Verification items for the finished model (mm, model axes). A direction names the side the tool comes from. Coordinates: 2 decimals unless noted, no trailing zeros. Loops run counter-clockwise (first coordinate to the right, second up) from the corner with the lowest first, then second, coordinate; pieces in that order, holes last. Notation, with made-up numbers: (-17.5, 19) - (-3.5, 19) arc R15 ccw to (-3.5, 23) - close; hole circle Ø6 at (20.25, 46.5). An arc over 180 degrees is marked (long way). One line per item, written item: value. Start each with the question number.
(1) Section check D-D (z = 0.5). Record the boundary of the cut face in (x, y).
(2) Gauge pin test, flat ends, axial feed: P1, Ø2.5, axis at x = 0, z = -12.75, coming from the +Y side; P2, Ø0.9, axis at x = 0, z = 12.75, coming from the +Y side; P3, Ø1.1, axis at x = -6.5, y = -0.5, coming from the +Z side; P4, Ø1.2, axis at y = -1, z = 9, coming from the -X side. Record the tip position at first contact, or that the pin passes through.
(3) Section check C-C (y = -0.9). Count the separate pieces of the cut face and the enclosed holes in it, plus the area to 3 significant figures.
(4) Section check B-B (x = 7.5). Record the boundary of the cut face in (y, z), plus the area to 3 significant figures.
(5) Set-up check for faces 5 (the face through (-4, 0, -9)), 6 (the face through (0, 0, -7.5)), 7 (the face through (5, -0.5, 0)): record each of +Z, -Z, +X, -X, +Y, -Y from which the full face is reachable in a straight line by a thin tool's end or side.
(6) Draft check along Z on faces 1 (the face through (0, 0, -11.5)), 2 (the face through (5, 0, -5)), 3 (the face through (9.859, -0.028, 2.797)), 4 (the face through (4, 0, -10)). Enter one of: +Z half, -Z half, draft (parallel to the pull), parting line (faces both ways), or undercut.
(7) Section check A-A (z = -10.75). Record the boundary of the cut face in (x, y), plus the area to 3 significant figures.
(8) Thickness scan on probe 1 along X at (y, z) = (-1, 0); probe 2 along X at (y, z) = (0.4, 0); probe 3 along X at (y, z) = (-0.2, 6.75). Record the ranges inside material, lowest first. Write a range as [from, to].
Autodesk Inventor part; units mm, degrees
ref_plane "YZ Plane" through (0, 0, 0) normal (1, 0, 0) x (0, 1, 0)
ref_plane "XZ Plane" through (0, 0, 0) normal (0, 1, 0) x (-1, 0, 0)
ref_plane "XY Plane" through (0, 0, 0) normal (0, 0, 1) x (1, 0, 0)
sketch "Sketch1" plane through (0, 0, 0) normal (0, 1, 0) x (-1, 0, 0)
  line L0 (4, -17) -> (-4, -17)
  line L1 (-4, -17) -> (-4, 0)
  line L2 (-4, 0) -> (4, 0)
  line L3 (4, 0) -> (4, -17)
  line L4 (4, -17) -> (-4, 0) construction
  line L5 (-4, -17) -> (4, 0) construction
  point P0 (0, 0)
  point P1 (0, -8.5)
  dimension "d0" = 8
  dimension "d1" = 17
  dimension "d19" = 0
  dimension "d20" = 0
extrude "Extrusion1" add sketch "Sketch1" along normal mid plane 4
sketch "Sketch2" plane through (0, 2, 0) normal (0, 1, 0) x (1, 0, 0)
  line L0 (-4, 17) -> (-4, 0)
  line L1 (-4, 0) -> (4, 0)
  line L2 (4, 0) -> (4, 17)
  line L3 (4, 17) -> (-4, 17)
  point P0 (0, 0)
  point P1 (0, 6.75)
  point P2 (0, 8.75)
  point P3 (0, 10.75)
  point P4 (0, 12.75)
  point P5 (0, 14.75)
  dimension "d4" = 6.75
  dimension "d7" = 2
hole "Hole1" at (0, 2, -6.75) at (0, 2, -8.75) at (0, 2, -10.75) at (0, 2, -12.75) at (0, 2, -14.75) direction (0, -1, 0) diameter 1.5 end through all
fillet "Fillet1" radius 4 2 edges at (-4, 0, -17) (4, 0, -17)
mirror "Mirror1" about plane through (0, 0, 0) normal (0, 0, 1) of "Extrusion1", "Hole1", "Fillet1"
sketch "Sketch3" plane through (0, 2, 0) normal (0, 1, 0) x (1, 0, 0)
  line L0 (11, -4) -> (4, -4)
  line L1 (4, -4) -> (4, 4)
  line L2 (4, 4) -> (11, 4)
  line L3 (11, 4) -> (11, -4)
  line L4 (11, -4) -> (4, 4) construction
  line L5 (4, -4) -> (11, 4) construction
  line L6 (4, 13) -> (4, -13)
  point P0 (0, 0)
  point P1 (7.5, 0)
  point P2 (4, -14)
  dimension "d22" = 0
  dimension "d23" = 0
  dimension "d24" = 8
  dimension "d25" = 7.5
extrude "Extrusion2" add sketch "Sketch3" against normal blind 4
fillet "Fillet2" radius 4 2 edges at (11, 0, -4) (11, 0, 4)
sketch "Sketch4" plane through (0, 2, 0) normal (0, 1, 0) x (1, 0, 0)
  point P0 (0, 0)
  point P1 (7.5, 0)
  dimension "d29" = 7.5
hole "Hole2" at (7.5, 2, 0) direction (0, -1, 0) diameter 4 end through all
mirror "Mirror2" about plane through (0, 0, 0) normal (1, 0, 0) of "Extrusion2", "Fillet2", "Hole2"
sketch "Sketch5" plane through (0, 2, 0) normal (0, 1, 0) x (1, 0, 0)
  circle A0 centre (0, 0) radius 3.75
  dimension "d37" = 7.5
extrude "Extrusion3" cut sketch "Sketch5" against normal through all
chamfer "Chamfer1" distance 2 angle 45 4 edges at (4, 0, 4) (-4, 0, 4) (-4, 0, -4) (4, 0, -4)
sketch "Sketch6" plane through (0, 2, 0) normal (0, 1, 0) x (1, 0, 0)
  circle A0 centre (0, 0) radius 3.75
  circle A1 centre (-7.5, 0) radius 2
  arc A2 (-7, 4) -> (-7, -4) centre (-7, 0) ccw
  line L0 (-6, -4) -> (-7, -4)
  line L1 (-4, -6) -> (-6, -4)
  line L2 (-4, -6) -> (-4, -13)
  arc A3 (-4, -13) -> (4, -13) centre (0, -13) ccw
  line L3 (4, -6) -> (4, -13)
  line L4 (6, -4) -> (4, -6)
  line L5 (6, -4) -> (7, -4)
  arc A4 (7, -4) -> (7, 4) centre (7, 0) ccw
  line L6 (7, 4) -> (6, 4)
  line L7 (4, 6) -> (6, 4)
  line L8 (4, 13) -> (4, 6)
  arc A5 (4, 13) -> (-4, 13) centre (0, 13) ccw
  line L9 (-4, 13) -> (-4, 6)
  line L10 (-6, 4) -> (-4, 6)
  line L11 (-7, 4) -> (-6, 4)
  circle A6 centre (7.5, 0) radius 2
  circle A7 centre (0, 12.75) radius 0.75
  circle A8 centre (0, 8.75) radius 0.75
  circle A9 centre (0, 6.75) radius 0.75
  circle A10 centre (0, 10.75) radius 0.75
  circle A11 centre (0, 14.75) radius 0.75
  circle A12 centre (0, -8.75) radius 0.75
  circle A13 centre (0, -6.75) radius 0.75
  circle A14 centre (0, -10.75) radius 0.75
  circle A15 centre (0, -14.75) radius 0.75
  circle A16 centre (0, -12.75) radius 0.75
  circle A17 centre (-7.5, 0) radius 3
  circle A18 centre (7.5, 0) radius 3
  dimension "d43" = 6
  dimension "d44" = 6
extrude "Extrusion4" cut sketch "Sketch6" against normal blind 2.5 contours A17 | A18
properties part number "JointPlate3"
Responses:
1. outline: (-10.97, -2) - (-9.44, -2) - (-9.44, -0.5) - (-10.46, -0.5) - (-10.46, 2) - (-10.97, 2) - close; (-5.56, -2) - (-3.72, -2) - (-3.72, 2) - (-4.54, 2) - (-4.54, -0.5) - (-5.56, -0.5) - close; (3.72, -2) - (5.56, -2) - (5.56, -0.5) - (4.54, -0.5) - (4.54, 2) - (3.72, 2) - close; (9.44, -2) - (10.97, -2) - (10.97, 2) - (10.46, 2) - (10.46, -0.5) - (9.44, -0.5) - close
2. P1: stops at y = 2
2. P2: passes through
2. P3: stops at z = 4.05
2. P4: stops at x = -4
3. separate pieces: 1
3. enclosed holes: 13
3. area: 278 mm²
4. outline: (-2, -3.97) - (2, -3.97) - (2, -3) - (-0.5, -3) - (-0.5, -2) - (-2, -2) - close; (-2, 2) - (-0.5, 2) - (-0.5, 3) - (2, 3) - (2, 3.97) - (-2, 3.97) - close
4. area: 10.7 mm²
5. face 5: -Z, -X, +Y, -Y
5. face 6: +Y, -Y
5. face 7: +Y
6. face 1: undercut
6. face 2: -Z half
6. face 3: +Z half
6. face 4: draft
7. outline: (-4, -2) - (-0.75, -2) - (-0.75, 2) - (-4, 2) - close; (0.75, -2) - (4, -2) - (4, 2) - (0.75, 2) - close
7. area: 26.0 mm²
8. probe 1: x = [-11, -9.5], [-5.5, -3.75], [3.75, 5.5], [9.5, 11]
8. probe 2: x = [-11, -10.5], [-4.5, -3.75], [3.75, 4.5], [10.5, 11]
8. probe 3: x = [-4, -0.75], [0.75, 4]
